from build123d import *

# Parameters (mm, degrees)
BOSS_EXTRUDE1_DEPTH = 127
SKETCH3_W           = 25.4
SKETCH3_H           = 25.4
CUT_EXTRUDE1_DEPTH  = 63.5
SKETCH4_R           = 10.16
CUT_EXTRUDE2_DEPTH  = 128.0000001


with BuildPart() as part:
    # Sketch2 → Boss-Extrude1 (new body)
    with BuildSketch(Plane(origin=(0, 0, 0), x_dir=(1, 0, 0), z_dir=(0, 1, 0))):
        with BuildLine():
            Line((0, 0), (127, 0))
            add(Edge.make_bspline(
                [(127, 0), (120.640280387, 68.469919386), (165.1, 126.964946797)],
                knots=[0, 0, 0, 1, 1, 1], degree=2))
            Line((165.1, 126.964946797), (-38.1, 126.964946797))
            add(Edge.make_bspline(
                [(0, 0), (6.359730642, 68.469923757), (-38.1, 126.964946797)],
                knots=[0, 0, 0, 1, 1, 1], degree=2))
        make_face()
    extrude(amount=-BOSS_EXTRUDE1_DEPTH)

    # Sketch3 → Cut-Extrude1 (cut)
    with BuildSketch(Plane.XY):
        with Locations((25.4, -25.4)):
            Rectangle(SKETCH3_W, SKETCH3_H)
        with Locations((25.4, -101.6)):
            Rectangle(SKETCH3_W, SKETCH3_H)
        with Locations((101.6, -25.4)):
            Rectangle(SKETCH3_W, SKETCH3_H)
        with Locations((101.6, -101.6)):
            Rectangle(SKETCH3_W, SKETCH3_H)
    extrude(amount=-CUT_EXTRUDE1_DEPTH, mode=Mode.SUBTRACT)

    # Sketch4 → Cut-Extrude2 (cut, through all)
    with BuildSketch(Plane(origin=(0, 0, 0), x_dir=(1, 0, 0), z_dir=(0, 1, 0))):
        with Locations((-12.447257457, 112.994946797)):
            Circle(SKETCH4_R)
        with Locations((139.447257457, 112.994946797)):
            Circle(SKETCH4_R)
    extrude(amount=-CUT_EXTRUDE2_DEPTH, mode=Mode.SUBTRACT)


solid = part.part
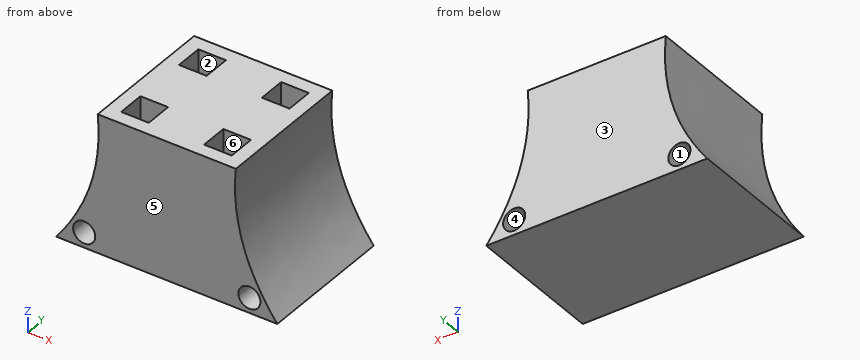
For this review, take the finished solid that the model builds, in its own axes (mm). Face numbers are marked on the shaded views. A direction names the side the tool comes from. Coordinates: 2 decimals unless noted, no trailing zeros. Answer as CSV lines item,"result". Start each with the question number.
1) Add section A-A (z = -56.5). Count the separate pieces of the cut face and the enclosed holes in it, then the cut area to 3 significant figures.
2) To check wall thickness, follow line 1 along Y through (x, z) = (17, -37); line 2 along X through (y, z) = (-22, -47.5); line 3 along X through (y, z) = (-20.5, -45). State the ranges of each line that lie inside material, in increasing order. Write a range as [from, to].
3) Draft analysis for pull direction Y (two halves, no side actions). For the marked faces 3, 4, 5 and 6, state which applies: +Y half, -Y half, draft (parallel to the pull), parting line (faces both ways), or undercut.
4) Insertion check: P1, Ø12, axis at y = -26, z = -92.5, coming from the -X side; P2, Ø12, axis at y = -61.5, z = -94, coming from the +X side. Each pin has a flat end and moves straight along its axis. Give the tip position at first contact, or say it passes through.
5) Machinability: for the marked faces 1 and 2, which of the approach directions +Z, -Z, +X, -X, +Y, -Y give a long, thin tool a straight path to every point of the face, cutting with its end or side? Answer none if there is none.
Result:
1,separate pieces,"1"
1,enclosed holes,"4"
1,area,"14,500 mm^2"
2,line 1,"[-127, -114.3], [-88.9, -38.1], [-12.7, 0]"
2,line 2,"[-1.91, 12.7], [38.1, 88.9], [114.3, 128.91]"
2,line 3,"[-1.48, 12.7], [38.1, 88.9], [114.3, 128.48]"
3,face 3,"+Y half"
3,face 4,"draft"
3,face 5,"-Y half"
3,face 6,"undercut"
4,P1,"x = -19.79"
4,P2,"x = 147.59"
5,face 1,"+Y, -Y"
5,face 2,"+Z"
